Here's how the part is built. I have some questions about the finished solid (model axes, mm). Coordinates: 2 decimals unless noted, no trailing zeros. Order: outer loops, then holes, each group sorted by start corner. A loop starts at its lowest first (then second) coordinate and runs counter-clockwise, first axis right, second up.
```python
from build123d import *

# Parameters (mm, degrees)
SKETCH1_R           = 1.4
BOSS_EXTRUDE1_DEPTH = 4


with BuildPart() as part:
    # Sketch1 → Boss-Extrude1 (new body)
    with BuildSketch(Plane.XY):
        with BuildLine():
            ThreePointArc((-11.000688459, -8.006682704), (-5.500688459, -13.506682704), (-0.000688459, -8.006682704))
            Line((-0.000688459, -8.006682704), (-0.000688459, 44.219898035))
            Line((-0.000688459, 44.219898035), (-0.000688459, 45.812285407))
            ThreePointArc((-0.000688459, 45.812285407), (-6.411717433, 51.067514262), (-12.077316081, 45.016091721))
            Line((-12.077316081, 45.016091721), (-12.072317389, 44.769911406))
            Line((-12.072317389, 44.769911406), (-11.000688459, -8.006682704))
        make_face()
        with Locations((-5.500688459, -8.006682704)):
            Circle(SKETCH1_R, mode=Mode.SUBTRACT)
        with Locations((-6.012756351, 45.016091721)):
            Circle(SKETCH1_R, mode=Mode.SUBTRACT)
    extrude(amount=BOSS_EXTRUDE1_DEPTH)


solid = part.part
```
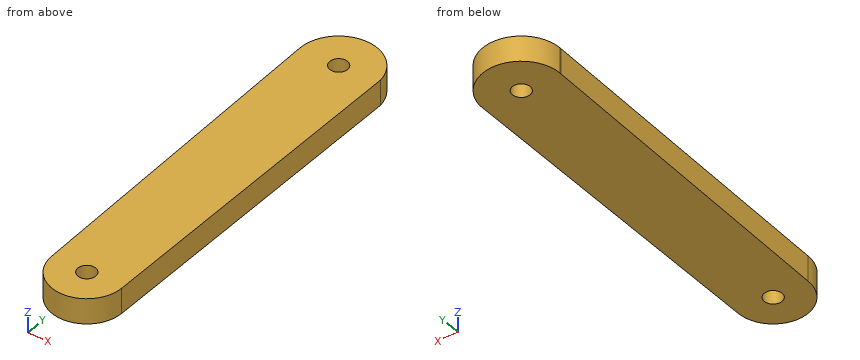
Q1. If we section it at B-B on x = -5.25: Write out the boundary of the cut face in (y, z), then the cut area to 3 significant figures.
Q2. I need wall thicknesses on L1, parallel to Y at x = -6, z = 1.45; L2, parallel to Y at x = -4.75, z = 2.4; L3, parallel to Y at x = -7, z = 3.45. Which ranges of each line are inside material? Lowest first, please.
Q3. If we section it at C-C on y = 36: Write out the boundary of the cut face in (x, z), then the cut area to 3 significant figures.
Q4. If we section it at D-D on x = -1.75: Write out the boundary of the cut face in (y, z), then the cut area to 3 significant figures.
Q5. If we section it at A-A on z = 1.5: Write out the boundary of the cut face in (x, y).
Q6. Will these pins go through, and if not, where does the flat tip stop? pin 1 (2 mm diameter, centred on y = 17.5, z = 3, fed in from -X); pin 2 (1 mm diameter, centred on x = -4.5, z = 3, fed in from +Y); pin 3 (1.5 mm diameter, centred on y = 25, z = 3.5, fed in from -X).
Reply:
1. outline: (-13.5, 0) - (-9.38, 0) - (-9.38, 4) - (-13.5, 4) - close; (-6.63, 0) - (43.84, 0) - (43.84, 4) - (-6.63, 4) - close; (46.19, 0) - (51.03, 0) - (51.03, 4) - (46.19, 4) - close
1. area: 238 mm2
2. L1: y = -13.48 to -9.31, -6.7 to 43.62, 46.42 to 51.08
2. L2: y = -13.46 to -9.19, -6.82 to 44.41, 45.62 to 50.95
2. L3: y = -13.3 to 44.02, 46.01 to 51
3. outline: (-11.89, 0) - (0, 0) - (0, 4) - (-11.89, 4) - close
3. area: 47.6 mm2
4. outline: (-12.03, 0) - (49.33, 0) - (49.33, 4) - (-12.03, 4) - close
4. area: 245 mm2
5. outline: (-12.08, 45.02) - (-11, -8.01) arc R5.5 ccw to (0, -8.01) - (0, 45.81) arc R6.06 ccw to start; hole circle Ø2.8 at (-6.01, 45.02); hole circle Ø2.8 at (-5.5, -8.01)
6. pin 1: stops at x = -11.54
6. pin 2: stops at y = 51
6. pin 3: stops at x = -11.69
